from build123d import *

# Parameters (mm, degrees)
EXTRUDE1_DEPTH     = 47.625
CUT_EXTRUDE1_DEPTH = 47.625
SKETCH3_R          = 5.1562
CUT_EXTRUDE2_DEPTH = 6.604
SKETCH4_R          = 3.175
CUT_EXTRUDE3_DEPTH = 10.4488
SKETCH5_R          = 2.0828
SKETCH5_R_2        = 3.2639
CUT_EXTRUDE4_DEPTH = 10.4488


with BuildPart() as part:
    # Sketch1 → Extrude1 (new body)
    with BuildSketch(Plane.XY):
        Polygon((55.524691805, 16.952365829), (55.524691805, 18.476365829), (61.730833978, 18.476365829), (61.729335279, 16.953119016), (70.543139545, 16.953119016), (71.305139176, 16.190369296), (71.305139176, 9.78956546), (70.543888896, 9.027565829), (19.685291805, 9.027565829), (18.923291805, 9.789565829), (18.923291805, 12.227965829), (19.685291805, 12.989965829), (41.961091805, 12.989965829), (45.923491805, 16.952365829), align=None)
    extrude(amount=EXTRUDE1_DEPTH)

    # Sketch2 → Cut-Extrude1 (cut)
    with BuildSketch(Plane.XZ.offset(-9.027565829)):
        with BuildLine():
            ThreePointArc((61.869039176, 36.5125), (60.913064999, 38.820425823), (58.605139176, 39.7764))
            Line((58.605139176, 39.7764), (58.605139176, 36.5125))
            Line((58.605139176, 36.5125), (61.869039176, 36.5125))
        make_face()
        with BuildLine():
            Line((58.605139176, 36.5125), (58.605139176, 39.7764))
            ThreePointArc((58.605139176, 39.7764), (56.297213353, 38.820425823), (55.341239176, 36.5125))
            Line((55.341239176, 36.5125), (58.605139176, 36.5125))
        make_face()
        with BuildLine():
            Line((61.869039176, 36.5125), (58.605139176, 36.5125))
            Line((58.605139176, 36.5125), (58.605139176, 33.2486))
            ThreePointArc((58.605139176, 33.2486), (60.913064999, 34.204574177), (61.869039176, 36.5125))
        make_face()
        with BuildLine():
            Line((58.605139176, 33.2486), (58.605139176, 36.5125))
            Line((58.605139176, 36.5125), (55.341239176, 36.5125))
            ThreePointArc((55.341239176, 36.5125), (56.297213353, 34.204574177), (58.605139176, 33.2486))
        make_face()
        with BuildLine():
            ThreePointArc((61.869039176, 11.1125), (60.913064999, 13.420425823), (58.605139176, 14.3764))
            Line((58.605139176, 14.3764), (58.605139176, 11.1125))
            Line((58.605139176, 11.1125), (61.869039176, 11.1125))
        make_face()
        with BuildLine():
            Line((58.605139176, 11.1125), (58.605139176, 14.3764))
            ThreePointArc((58.605139176, 14.3764), (56.297213353, 13.420425823), (55.341239176, 11.1125))
            Line((55.341239176, 11.1125), (58.605139176, 11.1125))
        make_face()
        with BuildLine():
            Line((61.869039176, 11.1125), (58.605139176, 11.1125))
            Line((58.605139176, 11.1125), (58.605139176, 7.8486))
            ThreePointArc((58.605139176, 7.8486), (60.913064999, 8.804574177), (61.869039176, 11.1125))
        make_face()
        with BuildLine():
            Line((58.605139176, 7.8486), (58.605139176, 11.1125))
            Line((58.605139176, 11.1125), (55.341239176, 11.1125))
            ThreePointArc((55.341239176, 11.1125), (56.297213353, 8.804574177), (58.605139176, 7.8486))
        make_face()
    extrude(amount=-CUT_EXTRUDE1_DEPTH, mode=Mode.SUBTRACT)

    # Sketch3 → Cut-Extrude2 (cut)
    with BuildSketch(Plane.XZ.offset(-9.027565829)):
        with Locations((58.605139176, 36.5125)):
            Circle(SKETCH3_R)
        with Locations((58.605139176, 11.1125)):
            Circle(SKETCH3_R)
    extrude(amount=-CUT_EXTRUDE2_DEPTH, mode=Mode.SUBTRACT)

    # Sketch4 → Cut-Extrude3 (cut, through all)
    with BuildSketch(Plane.XZ.offset(-9.027565829)):
        with Locations((45.905139176, 36.5125)):
            Circle(SKETCH4_R)
        with Locations((45.905139176, 11.1125)):
            Circle(SKETCH4_R)
    extrude(amount=-CUT_EXTRUDE3_DEPTH, mode=Mode.SUBTRACT)

    # Sketch5 → Cut-Extrude4 (cut, through all)
    with BuildSketch(Plane.XZ.offset(-9.027565829)):
        with Locations((29.014139176, 36.5125)):
            Circle(SKETCH5_R)
        with Locations((29.014139176, 11.1125)):
            Circle(SKETCH5_R)
        with Locations((29.014139176, 23.8125)):
            Circle(SKETCH5_R_2)
    extrude(amount=-CUT_EXTRUDE4_DEPTH, mode=Mode.SUBTRACT)


solid = part.part
Could you check a few things on this model? Use its own coordinates, in mm. A direction names the side the tool comes from. Give positions to 0.01 mm unless a question says otherwise; leave off trailing zeros. Write each loop counter-clockwise with the first axis right and the second up, starting at its lowest first coordinate (ties: lowest second). Pieces come first, ordered by that corner, then holes. Notation, with made-up numbers: (44, 58) -> (66, 58) arc R10 ccw to (66, 69) -> close; hole circle Ø3 at (19, 81). An arc over 180 degrees is marked (long way). Answer as CSV lines item,"result". Start each with the question number.
(1) Which directions (+Z, -Z, +X, -X, +Y, -Y) give clear straight access to the entire face, cutting with the end or side of a thin tool? Please do faces 4 (the face through (51, 16.952, 23)), 5 (the face through (66, 16.953, 23)), 6 (the face through (63.523, 12.283, 38.061)).
(2) If we section it at C-C, the plane y = 14.75: Give the number of separate pieces and of enclosed holes in the cut face, and give its area (3 significant figures).
(3) If we mould it in two halves opening along X, with no side actions, what happens to faces 1 (the face through (31, 10.98, 11.74)), 2 (the face through (71.305, 13, 23)), 3 (the face through (55.525, 18, 24))? For each: +X half, -X half, draft (parallel to the pull), parting line (faces both ways), or undercut.
(4) If we section it at D-D, the plane x = 60: Write out the boundary of the cut face in (y, z) (3 decimals).
(5) I'm going to push flat-ended pins straight in: pin 1 Ø4 at (x, z) = (45.91, 36.51) entering from +Y; pin 2 Ø8 at (x, z) = (58.61, 11.11) entering from -Y; pin 3 Ø1.2 at (y, z) = (18, 29.5) entering from -X; pin 4 Ø18 at (x, z) = (32, 28.5) entering from +Y. Where does each tip first touch, or does it pass through?
(6) If we section it at A-A, the plane x = 30: Write out the boundary of the cut face in (y, z) (3 decimals), and give its area (3 significant figures).
(7) Please list where these lines run through material, in increasing order: line 1 (Z direction, x = 28, y = 11.75) (3 decimals); line 2 (Z direction, x = 56, y = 10.5) (3 decimals); line 3 (Z direction, x = 60, y = 12.5) (3 decimals).
(8) If we section it at B-B, the plane z = 18: Write out the boundary of the cut face in (x, y), and give its area (3 significant figures).
Answer list:
1,face 4,"+Z, -Z, -X, +Y"
1,face 5,"+Z, -Z, +X, +Y"
1,face 6,"-Y"
2,separate pieces,"1"
2,enclosed holes,"2"
2,area,"1,090 mm^2"
3,face 1,"undercut"
3,face 2,"+X half"
3,face 3,"-X half"
4,outline,"(9.028, 0) -> (18.476, 0) -> (18.476, 8.162) -> (15.632, 8.162) -> (15.632, 6.149) -> (9.028, 6.149) -> close; (9.028, 16.076) -> (15.632, 16.076) -> (15.632, 14.063) -> (18.476, 14.063) -> (18.476, 33.562) -> (15.632, 33.562) -> (15.632, 31.549) -> (9.028, 31.549) -> close; (9.028, 41.476) -> (15.632, 41.476) -> (15.632, 39.463) -> (18.476, 39.463) -> (18.476, 47.625) -> (9.028, 47.625) -> close"
5,pin 1,"through"
5,pin 2,"y = 15.63"
5,pin 3,"x = 55.52"
5,pin 4,"y = 12.99"
6,outline,"(9.028, 0) -> (12.99, 0) -> (12.99, 9.278) -> (9.028, 9.278) -> close; (9.028, 12.947) -> (12.99, 12.947) -> (12.99, 20.701) -> (9.028, 20.701) -> close; (9.028, 26.924) -> (12.99, 26.924) -> (12.99, 34.678) -> (9.028, 34.678) -> close; (9.028, 38.347) -> (12.99, 38.347) -> (12.99, 47.625) -> (9.028, 47.625) -> close"
6,area,"135 mm^2"
7,line 1,"0 to 9.293, 12.932 to 20.71, 26.915 to 34.693, 38.332 to 47.625"
7,line 2,"0 to 6.663, 15.562 to 32.063, 40.962 to 47.625"
7,line 3,"0 to 6.149, 16.076 to 31.549, 41.476 to 47.625"
8,outline,"(18.92, 9.79) -> (19.69, 9.03) -> (70.54, 9.03) -> (71.31, 9.79) -> (71.31, 16.19) -> (70.54, 16.95) -> (61.73, 16.95) -> (61.73, 18.48) -> (55.52, 18.48) -> (55.52, 16.95) -> (45.92, 16.95) -> (41.96, 12.99) -> (19.69, 12.99) -> (18.92, 12.23) -> close"
8,area,"324 mm^2"
